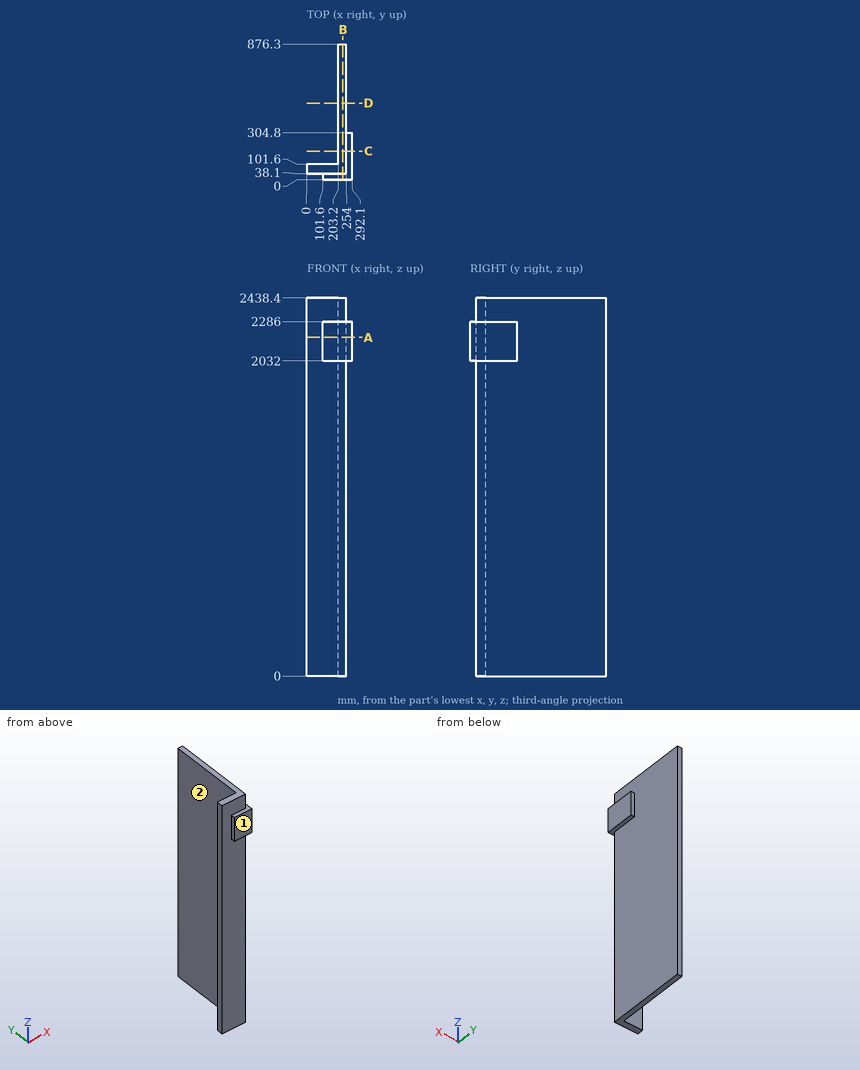
For this review, use the dimensioned drawing (mm, ordinates from the lowest corner) and the shaded views. A direction names the side the tool comes from. Round coordinates to 2 decimals unless told otherwise and drop trailing zeros. Write each loop counter-clockwise with the first axis right and the second up, starting at its lowest first coordinate (ties: lowest second). Pieces come first, ordered by that corner, then holes. Notation, with made-up numbers: (2, -2.5) - (14, -2.5) arc R23 ccw to (14, 17.5) - close; hole circle Ø8 at (-7.5, -18). An arc over 180 degrees is marked (long way). Answer as CSV lines item,"result". Start each with the question number.
(1) To check wall thickness, follow line 1 (Y direction, x = 41, z = 2201.5); line 2 (Y direction, x = 229, z = 1061); line 3 (X direction, y = 521.5, z = 758). State the ranges of each line that lie inside material, in increasing order.
(2) For pin 1 Ø5 at (y, z) = (599, 1360.5) entering from +X; pin 2 Ø8 at (x, z) = (160, 876) entering from -Y, all flat-tipped, find the tip position at first contact; note any pin that passes through.
(3) We need section C-C on y = 186. State the section outline as (x, z) points.
(4) We need section B-B on x = 232.5. State the section outline as (y, z) points.
(5) We need section A-A on z = 2184. State the section outline as (x, y) points.
(6) We need section D-D on y = 495.5. State the section outline as (x, z) points, plus the area to 3 significant figures.
(7) For the marked faces 1 and 2, list the 3-axis set-ups (+Z, -Z, +X, -X, +Y, -Y) from which the entire face can be reached by the end or side of a thin tool; tool diameter is ignored.
Worked answers:
1,line 1,"38.1 to 101.6"
1,line 2,"38.1 to 876.3"
1,line 3,"203.2 to 254"
2,pin 1,"x = 254"
2,pin 2,"y = 38.1"
3,outline,"(203.2, 0) - (254, 0) - (254, 2032) - (292.1, 2032) - (292.1, 2286) - (254, 2286) - (254, 2438.4) - (203.2, 2438.4) - close"
4,outline,"(0, 2032) - (38.1, 2032) - (38.1, 0) - (876.3, 0) - (876.3, 2438.4) - (38.1, 2438.4) - (38.1, 2286) - (0, 2286) - close"
5,outline,"(0, 38.1) - (101.6, 38.1) - (101.6, 0) - (292.1, 0) - (292.1, 304.8) - (254, 304.8) - (254, 876.3) - (203.2, 876.3) - (203.2, 101.6) - (0, 101.6) - close"
6,outline,"(203.2, 0) - (254, 0) - (254, 2438.4) - (203.2, 2438.4) - close"
6,area,"124,000 mm²"
7,face 1,"+Z, -Z, +X, -X, -Y"
7,face 2,"+Z, -Z, -X, +Y"
